For this review, take the finished solid that the model builds, in its own axes (mm). A direction names the side the tool comes from. Round coordinates to 2 decimals unless told otherwise and drop trailing zeros. Write each loop counter-clockwise with the first axis right and the second up, starting at its lowest first coordinate (ties: lowest second). Pieces come first, ordered by that corner, then holes. Notation, with made-up numbers: (-35.5, 48.5) -> (-24.5, 48.5) arc R17 ccw to (-24.5, 75.5) -> close; hole circle Ø11 at (63, 11.25). An arc over 180 degrees is marked (long way). Answer as CSV lines item,"result". Start each with the question number.
Item 1: Take a section at C-C on z = 7. Give the boundary of the cut face in (x, y).
Item 2: Wall thickness on probe 1 along Y at (x, z) = (0, 20); probe 2 along Z at (x, y) = (1, -26); probe 3 along X at (y, z) = (0.55, 13): over which ranges is each line inside the solid? List them lowest first. Write a range as from..to.
Item 3: Take a section at D-D on y = -16. Give the boundary of the cut face in (x, z).
Item 4: Take a section at A-A on x = 0. Give the boundary of the cut face in (y, z), then the cut area to 3 significant figures.
Item 5: Machinability: for faces 5 (the cylindrical face through (0, 29, 13)), 6 (the flat face through (-24.6, 2, 14.3)), 7 (the flat face through (24.6, -2, 14.3)), 8 (the flat face through (-24.6, -2, 14.3)), which of the approach directions +Z, -Z, +X, -X, +Y, -Y give a long, thin tool a straight path to every point of the face, cutting with its end or side? Answer none if there is none.
Item 6: For pin 1 Ø2.5 at (y, z) = (-26, 13) entering from -X; pin 2 Ø1 at (x, z) = (-6.5, 8.5) entering from -Y; pin 3 Ø1.8 at (y, z) = (25.5, 14) entering from +X; pin 4 Ø4 at (x, z) = (-26, 13) entering from -Y, all flat-tipped, find the tip position at first contact; note any pin that passes through.
Item 7: Mouldability with a two-part tool opening along Z and no side actions: class faces 1 (the cylindrical face through (0.028, 27.487, 13.195)), 2 (the cylindrical face through (29, 0, 13)), 3 (the cylindrical face through (-0.028, -27.487, 13.195)), 4 (the flat face through (24, 0, 16)) as +Z half, -Z half, draft (parallel to the pull), parting line (faces both ways), or undercut.
```python
from build123d import *

# Parameters (mm, degrees)
SKETCH_1_R               = 23
EXTRUDE_1_DEPTH          = 30
SKETCH_2_R               = 3
CUT_EXTRUDE_1_DEPTH      = 45.24929378
EXTRUDE_2_DEPTH          = 2
SKETCH_4_R               = 1.5
CUT_EXTRUDE_2_DEPTH      = 49.641546028
PATTERN_CIRCULAR_2_COUNT = 4


with BuildPart() as part:
    # Sketch 1 → Extrude 1 (new body)
    with BuildSketch(Plane.XY):
        Circle(SKETCH_1_R)
    extrude(amount=EXTRUDE_1_DEPTH)

    # Sketch 2 → Cut-Extrude 1 (cut, through all)
    with BuildSketch(Plane.XY.offset(30)):
        with Locations((16, 0)):
            Circle(SKETCH_2_R)
        with Locations((0, 16)):
            Circle(SKETCH_2_R)
        with Locations((-16, 0)):
            Circle(SKETCH_2_R)
        with Locations((0, -16)):
            Circle(SKETCH_2_R)
    extrude(amount=-CUT_EXTRUDE_1_DEPTH, mode=Mode.SUBTRACT)

    # Sketch 3 → Extrude 2 (add, symmetric)
    with BuildSketch(Plane(origin=(0, 0, 0), x_dir=(0, 0, -1), z_dir=(1, 0, 0))):
        with BuildLine():
            Line((-10, 22), (-16, 22))
            Line((-16, 22), (-16, 26))
            ThreePointArc((-16, 26), (-13, 29), (-10, 26))
            Line((-10, 26), (-10, 22))
        make_face()
    extrude_2 = extrude(amount=EXTRUDE_2_DEPTH, both=True)

    # Sketch 4 → Cut-Extrude 2 (cut, through all)
    with BuildSketch(Plane(origin=(2, 0, 0), x_dir=(0, 0, -1), z_dir=(1, 0, 0))):
        with Locations((-13, 26)):
            Circle(SKETCH_4_R)
    cut_extrude_2 = extrude(amount=-CUT_EXTRUDE_2_DEPTH, mode=Mode.SUBTRACT)

    # Pattern Circular 2: Extrude 2, Cut-Extrude 2 ×4 about axis
    pattern_circular_2_axis = Axis((0, 0, 0), (0, 0, 1))
    add([extrude_2.rotate(pattern_circular_2_axis, i * 360 / PATTERN_CIRCULAR_2_COUNT) for i in range(1, PATTERN_CIRCULAR_2_COUNT)])
    add([cut_extrude_2.rotate(pattern_circular_2_axis, i * 360 / PATTERN_CIRCULAR_2_COUNT) for i in range(1, PATTERN_CIRCULAR_2_COUNT)], mode=Mode.SUBTRACT)


solid = part.part
```
Output values:
1,outline,"circle Ø46 at (0, 0); hole circle Ø6 at (-16, 0); hole circle Ø6 at (0, -16); hole circle Ø6 at (0, 16); hole circle Ø6 at (16, 0)"
2,probe 1,"y = -23..-19, -13..13, 19..23"
2,probe 2,"z = 10..11.5, 14.5..16"
2,probe 3,"x = -29..-27.5, -24.5..-18.95, -13.05..13.05, 18.95..24.5, 27.5..29"
3,outline,"(-16.52, 0) -> (-3, 0) -> (-3, 30) -> (-16.52, 30) -> close; (3, 0) -> (16.52, 0) -> (16.52, 30) -> (3, 30) -> close"
4,outline,"(-26, 10) -> (-23, 10) -> (-23, 0) -> (-19, 0) -> (-19, 30) -> (-23, 30) -> (-23, 16) -> (-26, 16) arc R3 ccw to start; (-13, 0) -> (13, 0) -> (13, 30) -> (-13, 30) -> close; (19, 0) -> (23, 0) -> (23, 10) -> (26, 10) arc R3 ccw to (26, 16) -> (23, 16) -> (23, 30) -> (19, 30) -> close; hole circle Ø3 at (-26, 13); hole circle Ø3 at (26, 13)"
4,area,"1,070 mm^2"
5,face 5,"+X, -X, +Y"
5,face 6,"+Z, -Z, -X, +Y"
5,face 7,"+Z, -Z, +X, -Y"
5,face 8,"+Z, -Z, -X, -Y"
6,pin 1,"passes through"
6,pin 2,"stops at y = -22.2"
6,pin 3,"stops at x = 2"
6,pin 4,"stops at y = -2"
7,face 1,"undercut"
7,face 2,"parting line"
7,face 3,"undercut"
7,face 4,"+Z half"
